Job drawing, mm, ordinate dimensions from the low corner. One solid piece. Give positions to 0.01 mm unless a question says otherwise; leave off trailing zeros. Order: outer loops, then holes, each group sorted by start corner. A loop starts at its lowest first (then second) coordinate and runs counter-clockwise, first axis right, second up.
Item 1: Band-saw the part on A-A on y = 52. Give the cut face in (x, z).
Item 2: Band-saw the part on B-B on z = 89. Give the cut face in (x, y) (1 decimal).
Item 3: Wall check: L1, parallel to X at y = 35.5, z = 60; L2, parallel to X at y = 34.5, z = 95 (1 decimal); L3, parallel to Z at x = 86, y = 46 (1 decimal). Give the ranges that are in metal, low to high.
Item 4: Flat gauge pin, fed straight in: P1, Ø5, axis at x = 83.5, y = 52.5, coming from the +Z side (1 decimal). Where does the tip first touch, or does it go through?
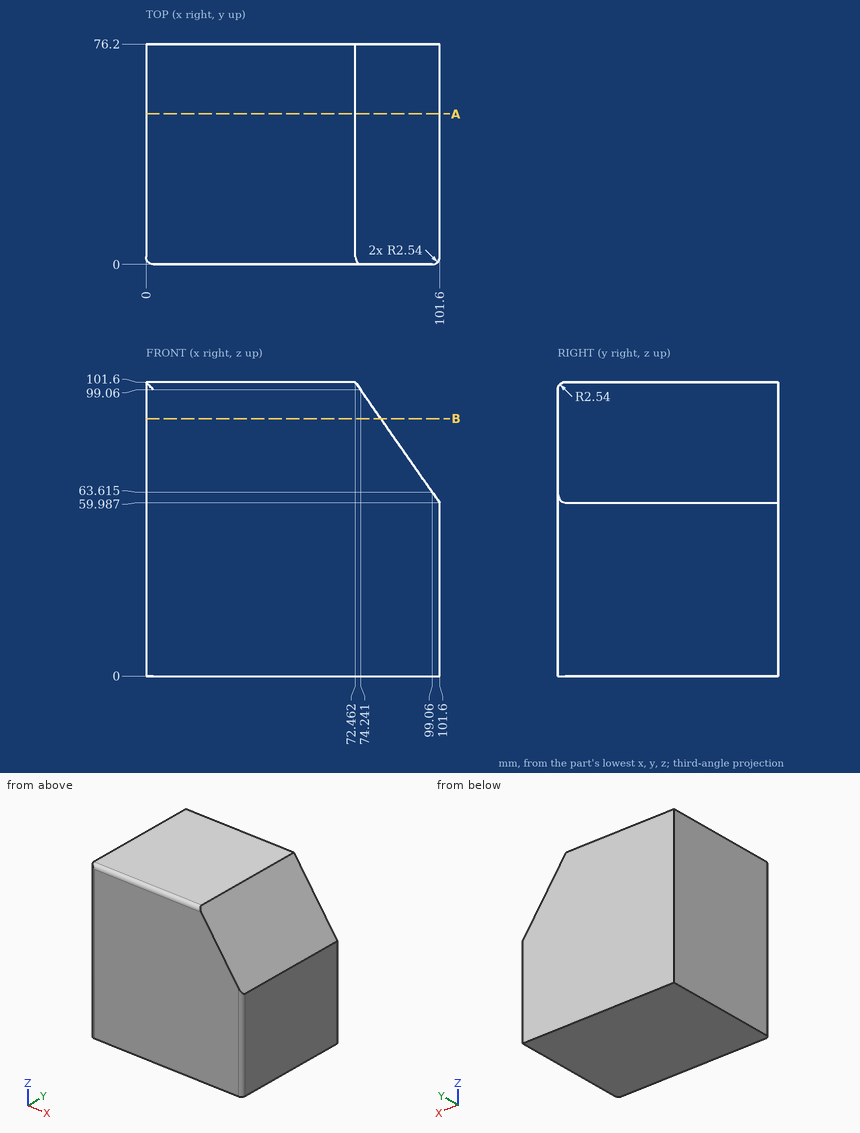
The answers:
1. outline: (0, 0) - (101.6, 0) - (101.6, 59.99) - (72.46, 101.6) - (0, 101.6) - close
2. outline: (0, 2.5) arc R2.5 ccw to (2.5, 0) - (81.3, 0) - (81.3, 76.2) - (0, 76.2) - close
3. L1: x = 0 to 101.59
3. L2: x = 0 to 77.1
3. L3: z = 0 to 82.3
4. P1: stops at z = 89.4
